Read the model definition and answer for the solid it produces. Units are mm, in the model's axes. A direction names the side the tool comes from. Coordinates: 2 decimals unless noted, no trailing zeros. Loops run counter-clockwise (first coordinate to the right, second up) from the corner with the lowest first, then second, coordinate; pieces in that order, holes last. Notation, with made-up numbers: M -27,16 L -17,16 A34 ccw -17,52 Z; hole C -15,4 d5. An arc over 180 degrees is marked long. One line per item, written item: value. Start each with the question number.
1. Flat-ended cylindrical pins translate along their axes: pin 1 (10 mm diameter, centred on x = -2, y = -6, fed in from +Z); pin 2 (1.5 mm diameter, centred on y = 4, z = 5, fed in from +X); pin 3 (10 mm diameter, centred on x = -0.5, y = -7, fed in from +Z); pin 4 (2 mm diameter, centred on y = -0.5, z = 4, fed in from +X). Find the tip coordinate at first contact, or state that the pin passes through.
2. The part is cut by section D-D (z = -0.25). Write down the section's boundary in (x, y).
3. The part is cut by section B-B (z = 1.5). Write down the section's boundary in (x, y).
4. Consider probe 1 along X at (y, z) = (-0.25, -0.5); probe 2 along X at (y, z) = (-0.75, 2.75); probe 3 along Z at (x, y) = (-0.25, 2.75). Determine where each line is inside the solid, lowest interval first.
5. For faces 5 (the face through (4.62, -0.02, 1.86)), 6 (the face through (0, 0, 0.254)), 7 (the face through (-0.05, -0.17, 5.8)), determine the directions among +Z, -Z, +X, -X, +Y, -Y from which every point of the face is accessible in a straight line to the end or side of a thin tool.
6. Determine the mould class of faces 1 (the face through (-3.691, 0, 5)), 2 (the face through (0.035, 0.022, 4.222)), 3 (the face through (-4.62, -0.02, 1.86)), 4 (the face through (3.691, 0, 1)) for opening direction Z: +Z half, -Z half, draft (parallel to the pull), parting line (faces both ways), or undercut.
```python
from build123d import *

# Parameters (mm, degrees)
SKETCH1_R               = 10.31875
BOSS_EXTRUDE1_DEPTH     = 0.79375
SKETCH5_W               = 9.525
SKETCH5_H               = 2.38125
BOSS_EXTRUDE2_DEPTH     = 0.254
BOSS_EXTRUDE3_DEPTH     = 2.38125
SKETCH7_R               = 1.5875
BOSS_EXTRUDE4_DEPTH     = 7.381946987
CUT_EXTRUDE1_DEPTH      = 17.513670686
CUT_EXTRUDE1_DEPTH_BACK = 17.513670686
SKETCH8_R               = 1.5875


with BuildPart() as part:
    # Sketch1 → Boss-Extrude1 (new body)
    with BuildSketch(Plane.XY):
        Circle(SKETCH1_R)
    extrude(amount=-BOSS_EXTRUDE1_DEPTH)

    # Sketch4 → Revolve1 (revolve)
    with BuildSketch(Plane(origin=(0, 0, 0), x_dir=(0, 0, -1), z_dir=(1, 0, 0))):
        with BuildLine():
            Line((0.79375, 0), (0.79375, 10.31875))
            ThreePointArc((0.79375, 10.31875), (1.982054014, 5.220075618), (2.38125, 0))
            Line((2.38125, 0), (0.79375, 0))
        make_face()
    revolve(axis=Axis((0, 0, -0.79375), (0, 0, -1)))

    # Sketch5 → Boss-Extrude2 (add)
    with BuildSketch(Plane.XY):
        Rectangle(SKETCH5_W, SKETCH5_H)
    extrude(amount=BOSS_EXTRUDE2_DEPTH)

    # Sketch6 → Boss-Extrude3 (add)
    with BuildSketch(Plane.XZ.offset(1.190625)):
        Polygon((-4.7625, 0.254), (-3.690973493, 0.254), (-3.690973493, 4.22275), (-4.484723493, 3.429), align=None)
        Polygon((4.7625, 0.254), (3.690973493, 0.254), (3.690973493, 4.22275), (4.484723493, 3.429), align=None)
    extrude(amount=-BOSS_EXTRUDE3_DEPTH)

    # Sketch7 → Boss-Extrude4 (add)
    with BuildSketch(Plane(origin=(-3.690973493, 0, 0), x_dir=(0, 0, -1), z_dir=(1, 0, 0))):
        with Locations(Location((-4.22275, 0, 0), (0, 0, 48.590377891))):
            Circle(SKETCH7_R)
    extrude(amount=BOSS_EXTRUDE4_DEPTH)

    # Sketch8 → Cut-Extrude1 (cut, two sides: drawn at the far end of the back side and taken through both)
    with BuildSketch(Plane.XZ.offset(1.190625).offset(-CUT_EXTRUDE1_DEPTH_BACK)):
        with Locations((0, 2.63525)):
            Circle(SKETCH8_R)
    extrude(amount=CUT_EXTRUDE1_DEPTH + CUT_EXTRUDE1_DEPTH_BACK, mode=Mode.SUBTRACT)


solid = part.part
```
Answer block:
1. pin 1: stops at z = 5.46
1. pin 2: passes through
1. pin 3: stops at z = 0
1. pin 4: stops at x = 4.52
2. outline: C 0,0 d20.64
3. outline: M -4.65,-1.19 L -3.69,-1.19 L -3.69,1.19 L -4.65,1.19 Z; M 3.69,-1.19 L 4.65,-1.19 L 4.65,1.19 L 3.69,1.19 Z
4. probe 1: x = -10.32 to 10.32
4. probe 2: x = -4.54 to -3.69, 3.69 to 4.54
4. probe 3: z = -2.27 to 0
5. face 5: +Z, +X, +Y, -Y
5. face 6: +Y, -Y
5. face 7: none
6. face 1: draft
6. face 2: undercut
6. face 3: +Z half
6. face 4: undercut
